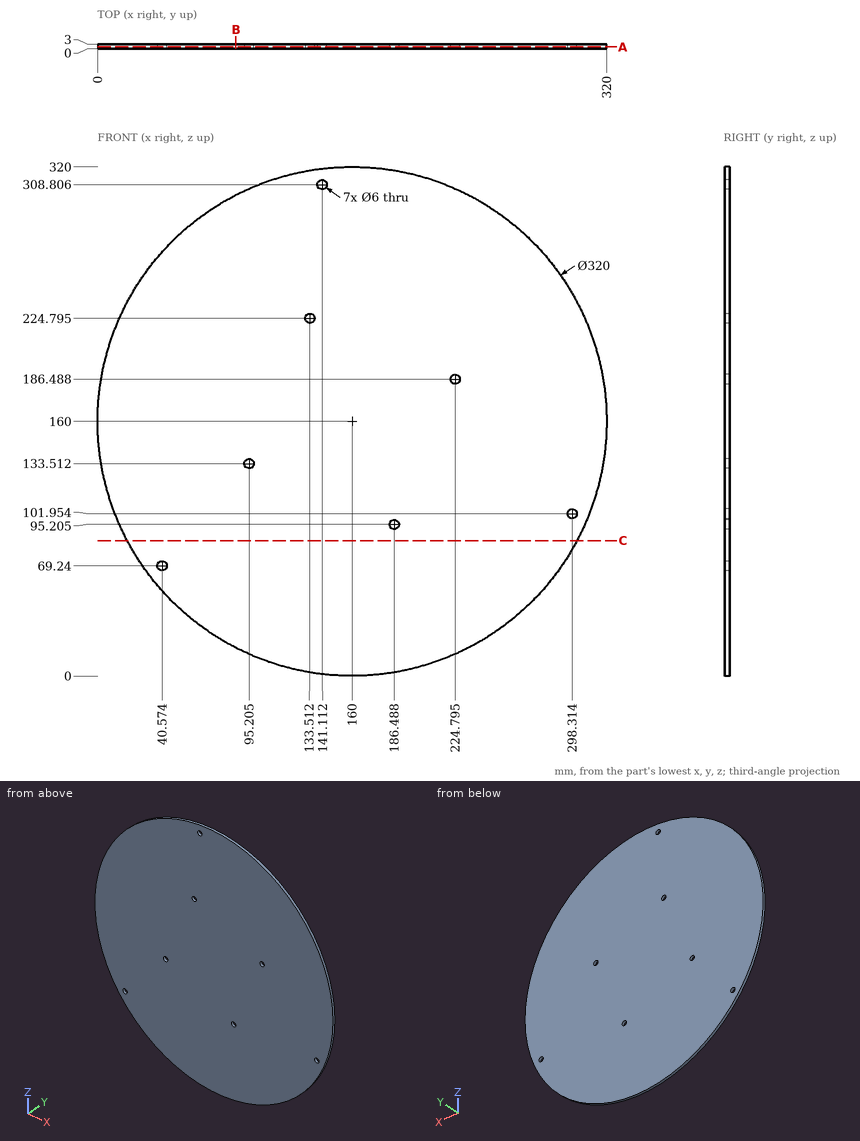
Part print with two shaded views. Sizes in mm from the minimum x, y, z corner. Coordinates: 2 decimals unless noted, no trailing zeros. Write each loop counter-clockwise with the first axis right and the second up, starting at its lowest first coordinate (ties: lowest second). Pieces come first, ordered by that corner, then holes. Notation, with made-up numbers: M 15,-26.75 L 52,-26.75 A24 cw 52,-16.75 Z; hole C 15,49.5 d11. An arc over 180 degrees is marked long. Return JSON: item names as keys, results as strings.
Item 1: Slice it at A-A, the plane y = 1.15. Write the cut outline in (x, z) (1 decimal).
Findings below:
{"outline": "C 160,160 d320; hole C 40.6,69.2 d6; hole C 95.2,133.5 d6; hole C 133.5,224.8 d6; hole C 141.1,308.8 d6; hole C 186.5,95.2 d6; hole C 224.8,186.5 d6; hole C 298.3,102 d6"}
Item 2: Probe line 1 (X direction, y = 0.9, z = 132.5); line 2 (Z direction, x = 224, y = 0.6) (1 decimal); line 3 (Z direction, x = 292.5, y = 1.4) (1 decimal). List the from-to ranges inside material, lowest first. Write a range as from..to.
Findings below:
{"line 1": "x = 2.38..92.38, 98.03..317.62", "line 2": "z = 13.4..183.6, 189.4..306.6", "line 3": "z = 70.3..249.7"}
Item 3: Slice it at C-C, the plane z = 85. Write the cut outline in (x, y).
Findings below:
{"outline": "M 18.67,0 L 301.33,0 L 301.33,3 L 18.67,3 Z"}
Item 4: Drop flat-ended pins along their axis: pin 1 Ø1.5 at (y, z) = (2.5, 213.5) entering from +X (1 decimal); pin 2 Ø3.5 at (x, z) = (141.11, 308.81) entering from +Y. Give the stop position or say it passes through.
Findings below:
{"pin 1": "stops at x = 311.1", "pin 2": "passes through"}
Item 5: Slice it at B-B, the plane x = 87. Write the cut outline in (y, z).
Findings below:
{"outline": "M 0,17.62 L 3,17.62 L 3,302.38 L 0,302.38 Z"}
